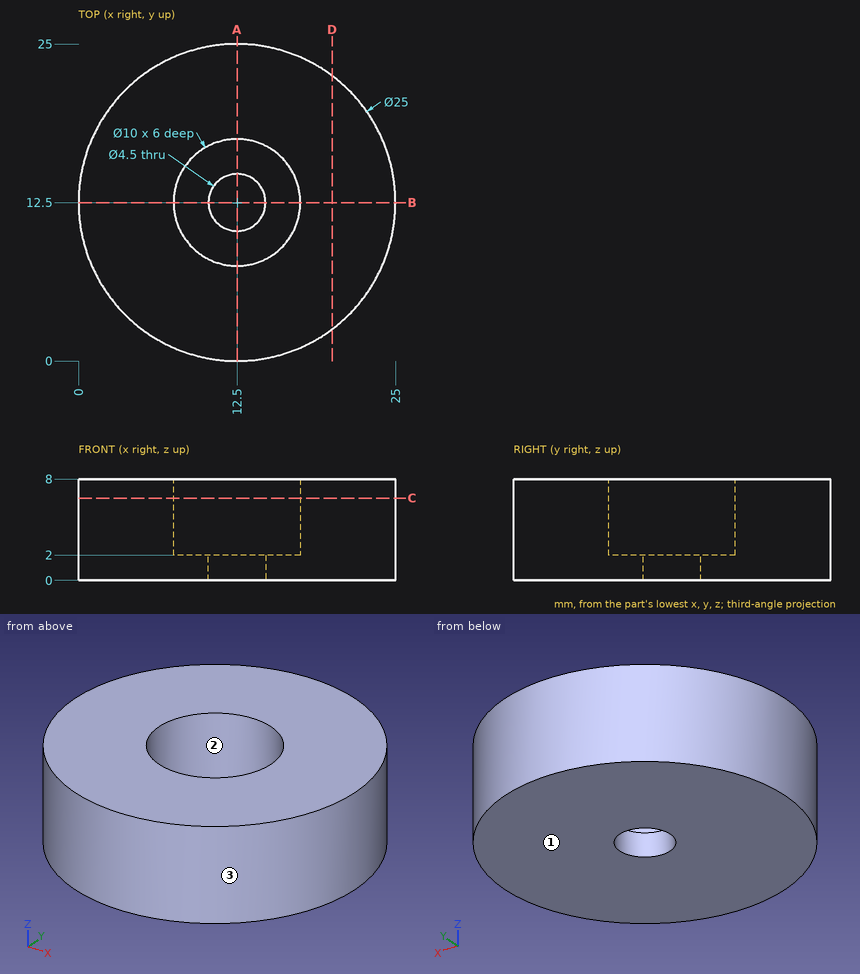
For this review, use the dimensioned drawing (mm, ordinates from the lowest corner) and the shaded views. Round coordinates to 2 decimals unless told otherwise and drop trailing zeros. Order: outer loops, then holes, each group sorted by start corner. A loop starts at its lowest first (then second) coordinate and runs counter-clockwise, first axis right, second up.
1) Consider section C-C (z = 6.5). State the section outline as (x, y) points.
The answers:
outline: circle Ø25 at (12.5, 12.5); hole circle Ø10 at (12.5, 12.5)
2) Draft analysis for pull direction X (two halves, no side actions). For the marked faces 1, 2 and 3, state which applies: released by +X, released by -X, zero draft, split by the parting line, or undercut.
The answers:
face 1: zero draft
face 2: undercut
face 3: split by the parting line
3) Consider section D-D (x = 20). State the section outline as (y, z) points.
The answers:
outline: (2.5, 0) - (22.5, 0) - (22.5, 8) - (2.5, 8) - close
4) Clearance check with flat-ended pins moving along their axes: pin 1 Ø2 at (y, z) = (20, 3.5) entering from +X; pin 2 Ø1.5 at (y, z) = (21, 2) entering from -X; pin 3 Ø1 at (x, y) = (15.5, 13.5) entering from +Z. State where each tip first meets the part, or that it passes through.
The answers:
pin 1: stops at x = 23.18
pin 2: stops at x = 2.69
pin 3: stops at z = 2
5) Consider section A-A (x = 12.5). State the section outline as (y, z) points, plus the area to 3 significant figures.
The answers:
outline: (0, 0) - (10.25, 0) - (10.25, 2) - (7.5, 2) - (7.5, 8) - (0, 8) - close; (14.75, 0) - (25, 0) - (25, 8) - (17.5, 8) - (17.5, 2) - (14.75, 2) - close
area: 131 mm2
6) For L1, parallel to Y at x = 12.5, z = 5.25; L2, parallel to Y at x = 12.5, z = 0.65; L3, parallel to Z at x = 12.5, y = 17, list the stretches that pass through material, from the lowest coordinate up.
The answers:
L1: y = 0 to 7.5, 17.5 to 25
L2: y = 0 to 10.25, 14.75 to 25
L3: z = 0 to 2
